Design review of the part built by this model. Coordinates are the model's own, in mm. Round coordinates to 2 decimals unless told otherwise and drop trailing zeros. Loops run counter-clockwise (first coordinate to the right, second up) from the corner with the lowest first, then second, coordinate; pieces in that order, holes last. Notation, with made-up numbers: (-2.75, 8.25) -> (11.25, 8.25) arc R23 cw to (11.25, 31.25) -> close; hole circle Ø4 at (81.5, 61.5). An arc over 180 degrees is marked (long way). Answer as CSV lines item,"result". Start each with the question number.
(1) Take a section at A-A, the plane x = 60. Write out the cut boundary in (y, z), and give its area (3 significant figures).
(2) Take a section at B-B, the plane y = 1.1. State how many separate pieces and enclosed holes the cut face has, and give its area (3 significant figures).
(3) To check wall thickness, follow line 1 (X direction, y = 2.7, z = 35); line 2 (X direction, y = 1.65, z = 0); line 3 (X direction, y = 2.35, z = -0.5). State the ranges of each line that lie inside material, in increasing order. Write a range as from..to.
(4) Take a section at D-D, the plane z = 0. Write out the cut boundary in (x, y).
(5) Take a section at C-C, the plane z = -26. Write out the cut boundary in (x, y), and give its area (3 significant figures).
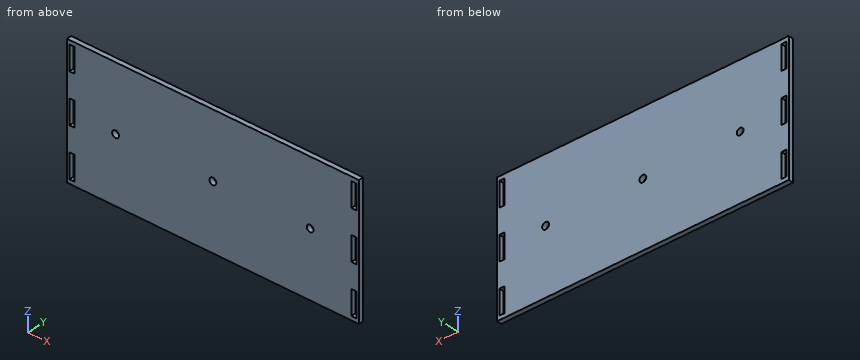
from build123d import *

# Parameters (mm, degrees)
SKETCH_1_W      = 180
SKETCH_1_H      = 80
SKETCH_1_R      = 2.1
SKETCH_1_W_2    = 3.05
SKETCH_1_H_2    = 15
EXTRUDE_1_DEPTH = 3


with BuildPart() as part:
    # 草图1 → 凸台-拉伸1 (new body)
    with BuildSketch(Plane(origin=(0, 0, 0), x_dir=(1, 0, 0), z_dir=(0, 1, 0))):
        Rectangle(SKETCH_1_W, SKETCH_1_H)
        with Locations(Location((-60, 0, 0), (0, 0, 270))):
            Circle(SKETCH_1_R, mode=Mode.SUBTRACT)
        with Locations(Location((0, 0, 0), (0, 0, 270))):
            Circle(SKETCH_1_R, mode=Mode.SUBTRACT)
        with Locations(Location((60, 0, 0), (0, 0, 270))):
            Circle(SKETCH_1_R, mode=Mode.SUBTRACT)
        with Locations((-86.975, 30)):
            Rectangle(SKETCH_1_W_2, SKETCH_1_H_2, mode=Mode.SUBTRACT)
        with Locations((-86.975, 0)):
            Rectangle(SKETCH_1_W_2, SKETCH_1_H_2, mode=Mode.SUBTRACT)
        with Locations((-86.975, -30)):
            Rectangle(SKETCH_1_W_2, SKETCH_1_H_2, mode=Mode.SUBTRACT)
        with Locations((86.975, 30)):
            Rectangle(SKETCH_1_W_2, SKETCH_1_H_2, mode=Mode.SUBTRACT)
        with Locations((86.975, -30)):
            Rectangle(SKETCH_1_W_2, SKETCH_1_H_2, mode=Mode.SUBTRACT)
        with Locations((86.975, 0)):
            Rectangle(SKETCH_1_W_2, SKETCH_1_H_2, mode=Mode.SUBTRACT)
    extrude(amount=EXTRUDE_1_DEPTH)


solid = part.part
The answers:
1,outline,"(0, -40) -> (3, -40) -> (3, -2.1) -> (0, -2.1) -> close; (0, 2.1) -> (3, 2.1) -> (3, 40) -> (0, 40) -> close"
1,area,"227 mm²"
2,separate pieces,"1"
2,enclosed holes,"9"
2,area,"14,100 mm²"
3,line 1,"-90..-88.5, -85.45..85.45, 88.5..90"
3,line 2,"-90..-88.5, -85.45..-62.1, -57.9..-2.1, 2.1..57.9, 62.1..85.45, 88.5..90"
3,line 3,"-90..-88.5, -85.45..-62.04, -57.96..-2.04, 2.04..57.96, 62.04..85.45, 88.5..90"
4,outline,"(-90, 0) -> (-88.5, 0) -> (-88.5, 3) -> (-90, 3) -> close; (-85.45, 0) -> (-62.1, 0) -> (-62.1, 3) -> (-85.45, 3) -> close; (-57.9, 0) -> (-2.1, 0) -> (-2.1, 3) -> (-57.9, 3) -> close; (2.1, 0) -> (57.9, 0) -> (57.9, 3) -> (2.1, 3) -> close; (62.1, 0) -> (85.45, 0) -> (85.45, 3) -> (62.1, 3) -> close; (88.5, 0) -> (90, 0) -> (90, 3) -> (88.5, 3) -> close"
5,outline,"(-90, 0) -> (-88.5, 0) -> (-88.5, 3) -> (-90, 3) -> close; (-85.45, 0) -> (85.45, 0) -> (85.45, 3) -> (-85.45, 3) -> close; (88.5, 0) -> (90, 0) -> (90, 3) -> (88.5, 3) -> close"
5,area,"522 mm²"
